```python
from build123d import *

# Parameters (mm, degrees)
ESBO_O1_W                = 82.8
ESBO_O1_H                = 34.8
RESSALTO_EXTRUS_O1_DEPTH = 4
CASCA2_T                 = 0.4
ESBO_O2_W                = 79.6
ESBO_O2_H                = 31.6
ESBO_O2_W_2              = 78.8
ESBO_O2_H_2              = 30.8
RESSALTO_EXTRUS_O2_DEPTH = 4
FILETE1_R                = 1


with BuildPart() as part:
    # Esboço1 → Ressalto-extrusão1 (new body)
    with BuildSketch(Plane(origin=(0, 0, 0), x_dir=(1, 0, 0), z_dir=(0, 1, 0))):
        Rectangle(ESBO_O1_W, ESBO_O1_H)
    extrude(amount=RESSALTO_EXTRUS_O1_DEPTH)

    # Casca2
    casca2_openings = [part.faces().sort_by_distance(p)[0] for p in [
        (0, 4, 0),
    ]]
    offset(amount=CASCA2_T, openings=casca2_openings, kind=Kind.INTERSECTION)

    # Esboço2 → Ressalto-extrusão2 (add)
    with BuildSketch(Plane(origin=(0, 0, 0), x_dir=(1, 0, 0), z_dir=(0, 1, 0))):
        Rectangle(ESBO_O2_W, ESBO_O2_H)
        Rectangle(ESBO_O2_W_2, ESBO_O2_H_2, mode=Mode.SUBTRACT)
    extrude(amount=RESSALTO_EXTRUS_O2_DEPTH)

    # Filete1
    filete1_edges = [part.edges().sort_by_distance(p)[0] for p in [
        (-41.4, 2, -17.4),
        (-41.4, 2, 17.4),
        (41.4, 2, 17.4),
        (41.4, 2, -17.4),
        (39.8, 2, -15.8),
        (-39.8, 2, -15.8),
        (-39.8, 2, 15.8),
        (39.8, 2, 15.8),
        (-39.4, 2, -15.4),
        (-39.4, 2, 15.4),
        (39.4, 2, 15.4),
        (39.4, 2, -15.4),
        (-41.8, 1.8, -17.8),
        (41.8, 1.8, -17.8),
        (41.8, 1.8, 17.8),
        (-41.8, 1.8, 17.8),
    ]]
    fillet(filete1_edges, radius=FILETE1_R)


solid = part.part
```
Build history of the part. All positions in model axes, mm. A direction names the side the tool comes from. Coordinates: 2 decimals unless noted, no trailing zeros. Order: outer loops, then holes, each group sorted by start corner. A loop starts at its lowest first (then second) coordinate and runs counter-clockwise, first axis right, second up. Notation, with made-up numbers: M 42,39.5 L 92,39.5 A9 ccw 92,49.5 Z; hole C 34.25,-0.5 d7. An arc over 180 degrees is marked long. One line per question, with ' | ' between items. Start each with the question number.
1. Mould opens along X. For faces 1 (the face through (-1, 2, 17.8)), 2 (the face through (41.8, 2, 0)), 3 (the face through (-1, 2, -15.8)) say: +X half, -X half, draft (parallel to the pull), parting line (faces both ways), or undercut.
2. Flat gauge pin, fed straight in: P1, Ø10.5, axis at x = -19.5, z = 6, coming from the +Y side. Where does the tip first touch, or does it go through?
3. Cut at C-C (z = 9). Write the cut outline in (x, y), plus the area to 3 significant figures.
4. Cut at A-A (y = 2.45). Count the separate pieces of the cut face and the enclosed holes in it, plus the area to 3 significant figures.
5. Wall check: line 1 along X through (y, z) = (2.25, -14.5); line 2 along Z through (x, y) = (-21, 1.05); line 3 along Y through (x, z) = (10, -6). Give the ranges that are in metal, low to high. Write a range as [from, to].
6. Cut at B-B (x = 31.5). Write the cut outline in (y, z).
7. Tool access for faces 4 (the face through (-1, 2, 15.4)), 5 (the face through (-1, 2, -17.8)): list every direction of +Z, -Z, +X, -X, +Y, -Y with a clear straight run to the whole face (end or side of a thin tool).
The answers:
1) face 1: draft | face 2: +X half | face 3: undercut
2) P1: stops at y = 0
3) outline: M -41.8,-0.4 L 41.8,-0.4 L 41.8,4 L 41.4,4 L 41.4,0 L 39.8,0 L 39.8,4 L 39.4,4 L 39.4,0 L -39.4,0 L -39.4,4 L -39.8,4 L -39.8,0 L -41.4,0 L -41.4,4 L -41.8,4 Z | area: 39.8 mm2
4) separate pieces: 2 | enclosed holes: 2 | area: 183 mm2
5) line 1: x = [-41.8, -41.4], [-39.8, -39.39], [39.39, 39.8], [41.4, 41.8] | line 2: z = [-17.8, -17.4], [-15.8, -15.4], [15.4, 15.8], [17.4, 17.8] | line 3: y = [-0.4, 0]
6) outline: M -0.4,-17.8 L 4,-17.8 L 4,-17.4 L 0,-17.4 L 0,-15.8 L 4,-15.8 L 4,-15.4 L 0,-15.4 L 0,15.4 L 4,15.4 L 4,15.8 L 0,15.8 L 0,17.4 L 4,17.4 L 4,17.8 L -0.4,17.8 Z
7) face 4: +Y | face 5: -Z, +X, -X, +Y, -Y
